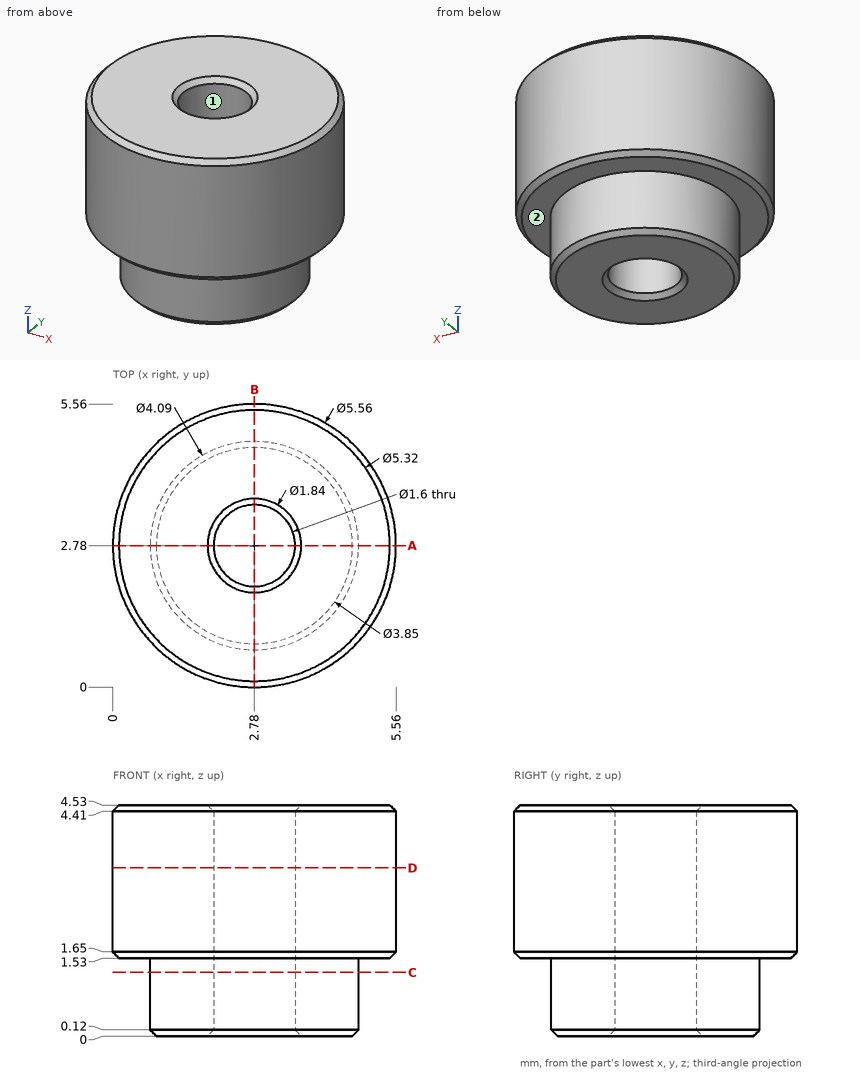
Verification items for this drawing (mm, ordinates from the low corner). A direction names the side the tool comes from. Give positions to 0.01 mm unless a question says otherwise; leave off trailing zeros. Loops run counter-clockwise (first coordinate to the right, second up) from the corner with the lowest first, then second, coordinate; pieces in that order, holes last. Notation, with made-up numbers: M 24.5,31.5 L 62.5,31.5 A20 ccw 62.5,35.5 Z; hole C 17.25,84.5 d2. An arc over 180 degrees is marked long. Write each question's results on one line, items separated by ' | '.
1) Tool access check on the marked faces 1 and 2. Record the directions out of +Z, -Z, +X, -X, +Y, -Y that give a thin tool (end or side, any length) a straight path to the whole face; none if there is none.
Answers follow:
face 1: +Z, -Z | face 2: -Z
2) Section check A-A, the plane y = 2.78. Record the boundary of the cut face in (x, z) (3 decimals), plus the area to 3 significant figures.
Answers follow:
outline: M 0,1.65 L 0.12,1.53 L 0.735,1.53 L 0.735,0.12 L 0.855,0 L 1.86,0 L 1.98,0.12 L 1.98,4.41 L 1.86,4.53 L 0.12,4.53 L 0,4.41 Z; M 3.58,0.12 L 3.7,0 L 4.705,0 L 4.825,0.12 L 4.825,1.53 L 5.44,1.53 L 5.56,1.65 L 5.56,4.41 L 5.44,4.53 L 3.7,4.53 L 3.58,4.41 Z | area: 15.6 mm2
3) Gauge pin test, flat ends, axial feed: pin 1 (1 mm diameter, centred on y = 1, z = 1, fed in from +X); pin 2 (3 mm diameter, centred on x = 1, y = 4, fed in from -Z); pin 3 (1 mm diameter, centred on x = 5, z = 3.5, fed in from +Y). Record the tip position at first contact, or that the pin passes through.
Answers follow:
pin 1: x = 4.37 | pin 2: z = 0 | pin 3: y = 4.96
4) Thickness scan on line 1 (Y direction, x = 2.78, z = 3.55); line 2 (Y direction, x = 2.78, z = 1.15) (3 decimals); line 3 (Z direction, x = 0.55, y = 3.6). Record the ranges inside material, lowest first.
Answers follow:
line 1: 0 to 1.98, 3.58 to 5.56 | line 2: 0.735 to 1.98, 3.58 to 4.825 | line 3: 1.53 to 4.53
5) Section check C-C, the plane z = 1.25. Record the boundary of the cut face in (x, y) (3 decimals).
Answers follow:
outline: C 2.78,2.78 d4.09; hole C 2.78,2.78 d1.6
6) Section check D-D, the plane z = 3.3. Record the boundary of the cut face in (x, y).
Answers follow:
outline: C 2.78,2.78 d5.56; hole C 2.78,2.78 d1.6
